from build123d import *

# Parameters (mm, degrees)
CUT_EXTRUDE1_DEPTH = 50
CUT_EXTRUDE2_DEPTH = 50


with BuildPart() as part:
    # Sketch1 → Revolve1 (revolve)
    with BuildSketch(Plane.XY):
        Polygon((11.25, 10.82996466), (11.25, -1.17003534), (22.5, -1.17003534), (31.753664233, 40.82996466), (25.609760166, 40.82996466), (19, 10.82996466), align=None)
    revolve(axis=Axis((0, 29.136855034, 0), (0, -1, 0)))

    # Sketch2 → Cut-Extrude1 (cut, symmetric)
    with BuildSketch(Plane(origin=(0, 0, 0), x_dir=(0, 0, -1), z_dir=(1, 0, 0))):
        with BuildLine():
            Line((-3.547836686, 40.82996466), (3.547836686, 40.82996466))
            ThreePointArc((3.547836686, 40.82996466), (0, 37.282127974), (-3.547836686, 40.82996466))
        make_face()
    extrude(amount=CUT_EXTRUDE1_DEPTH, both=True, mode=Mode.SUBTRACT)

    # Sketch3 → Cut-Extrude2 (cut, symmetric)
    with BuildSketch(Plane.XY):
        with BuildLine():
            Line((-2.456970945, 40.82996466), (2.456970945, 40.82996466))
            ThreePointArc((2.456970945, 40.82996466), (0, 38.372993715), (-2.456970945, 40.82996466))
        make_face()
    extrude(amount=CUT_EXTRUDE2_DEPTH, both=True, mode=Mode.SUBTRACT)


solid = part.part
The model under review builds one solid part; all positions refer to its coordinate system, in mm. A direction names the side the tool comes from. Give positions to 0.01 mm unless a question says otherwise; leave off trailing zeros. Order: outer loops, then holes, each group sorted by start corner. A loop starts at its lowest first (then second) coordinate and runs counter-clockwise, first axis right, second up. Notation, with made-up numbers: M -29,44.5 L 28,44.5 A19 cw 28,64.5 Z; hole C 12.5,51.25 d7. An arc over 180 degrees is marked long. One line per question, with ' | ' between items. Start each with the question number.
1) Consider section A-A, the plane x = 0. Give the boundary of the cut face in (y, z), then the cut area to 3 significant figures.
2) For faces 4 (the face through (-19, 40.83, -19)), 5 (the face through (8.2, 10.83, -8.2)), list the 3-axis set-ups (+Z, -Z, +X, -X, +Y, -Y) from which the entire face can be reached by the end or side of a thin tool; tool diameter is ignored.
3) Clearance check with flat-ended pins moving along their axes: P1, Ø8, axis at x = -21, y = 3.5, coming from the +Z side; P2, Ø3, axis at x = 17.5, y = 6, coming from the -Z side; P3, Ø20, axis at x = 0, z = 0, coming from the +Y side; P4, Ø1.5, axis at x = -17.5, y = 29, coming from the +Z side. State where each tip first meets the part, or that it passes through.
4) Consider section C-C, the plane y = 35. Give the boundary of the cut face in (x, z).
5) Mouldability with a two-part tool opening along X and no side actions: class faces 1 (the face through (5.3, -1.17, 10.3)), 2 (the face through (24.955, 15.457, 7.859)), 3 (the face through (0.054, 38.374, 28.41)) as pulls with the +X half, pulls with the -X half, needs draft (parallel to the pull), parting line crosses it, or undercut.
6) Wall thickness on L1, parallel to Z at x = 0, y = 6.5; L2, parallel to Z at x = 0, y = 1; L3, parallel to X at y = 26.5, z = -14.5: over which ranges is each line inside the solid? List them lowest first. Write a range as from..to.
7) Consider section B-B, the plane z = 0. Give the boundary of the cut face in (x, y).
Found:
1) outline: M -1.17,-22.5 L 38.37,-31.21 L 38.37,-25.07 L 10.83,-19 L 10.83,-11.25 L -1.17,-11.25 Z; M -1.17,11.25 L 10.83,11.25 L 10.83,19 L 38.37,25.07 L 38.37,31.21 L -1.17,22.5 Z | area: 640 mm²
2) face 4: +Z, -Z, +X, -X, +Y | face 5: +Y
3) P1: stops at z = 16.46 | P2: stops at z = -18.07 | P3: passes through | P4: stops at z = 23.89
4) outline: C 0,0 d60.94; hole C 0,0 d48.65
5) face 1: needs draft | face 2: parting line crosses it | face 3: undercut
6) L1: z = -24.19..-11.25, 11.25..24.19 | L2: z = -22.98..-11.25, 11.25..22.98 | L3: x = -24.65..-17.14, 17.14..24.65
7) outline: M -30.97,37.28 L -22.5,-1.17 L -11.25,-1.17 L -11.25,10.83 L -19,10.83 L -24.83,37.28 Z; M 11.25,-1.17 L 22.5,-1.17 L 30.97,37.28 L 24.83,37.28 L 19,10.83 L 11.25,10.83 Z
